Input: part model. Units: mm. Frame: model coordinates. A direction names the side the tool comes from. Round coordinates to 2 decimals unless told otherwise and drop trailing zeros. Write each loop counter-clockwise with the first axis right and the second up, starting at its lowest first coordinate (ties: lowest second). Pieces come first, ordered by that corner, then holes. Notation, with made-up numbers: (39, 87) - (96, 87) arc R15 cw to (96, 91) - close; hole circle Ø11 at (-31.75, 56.25). An arc over 180 degrees is marked (long way). Use one line per item in the form item = value.
```python
from build123d import *

# Parameters (mm, degrees)
SKETCH1_R             = 5
BOSS_EXTRUDE1_DEPTH   = 0.1
BOSS_EXTRUDE1_2_DEPTH = 0.1
BOSS_EXTRUDE1_3_DEPTH = 0.1
BOSS_EXTRUDE1_4_DEPTH = 0.1
BOSS_EXTRUDE2_DEPTH   = 3


with BuildPart() as part:
    # Sketch1 → Boss-Extrude1 (new body)
    with BuildSketch(Plane.XY):
        with Locations((-44.491847198, 44.491847198)):
            Circle(SKETCH1_R)
    extrude(amount=BOSS_EXTRUDE1_DEPTH)



with BuildPart() as body_2:
    # Sketch1 → Boss-Extrude1 2 (new body)
    with BuildSketch(Plane.XY):
        with Locations((44.491847198, 44.491847198)):
            Circle(SKETCH1_R)
    extrude(amount=BOSS_EXTRUDE1_2_DEPTH)


with BuildPart() as body_3:
    # Sketch1 → Boss-Extrude1 3 (new body)
    with BuildSketch(Plane.XY):
        with Locations((44.491847198, -44.491847198)):
            Circle(SKETCH1_R)
    extrude(amount=BOSS_EXTRUDE1_3_DEPTH)


with BuildPart() as body_4:
    # Sketch1 → Boss-Extrude1 4 (new body)
    with BuildSketch(Plane.XY):
        with Locations((-44.491847198, -44.491847198)):
            Circle(SKETCH1_R)
    extrude(amount=BOSS_EXTRUDE1_4_DEPTH)


with BuildPart() as part_1:
    add(part.part)

    add(body_2.part)  # Boss-Extrude2 merges body 2

    add(body_3.part)  # Boss-Extrude2 merges body 3

    add(body_4.part)  # Boss-Extrude2 merges body 4
    # Sketch2 → Boss-Extrude2 (add)
    with BuildSketch(Plane.XY):
        with BuildLine():
            Line((-59.341089603, 40.956313292), (-40.956313292, 59.341089603))
            ThreePointArc((-40.956313292, 59.341089603), (0, 47.170862812), (40.956313292, 59.341089603))
            Line((40.956313292, 59.341089603), (59.341089603, 40.956313292))
            ThreePointArc((59.341089603, 40.956313292), (39.686643359, 0), (59.341089603, -40.956313292))
            Line((59.341089603, -40.956313292), (40.956313292, -59.341089603))
            ThreePointArc((40.956313292, -59.341089603), (0, -47.170862812), (-40.956313292, -59.341089603))
            Line((-40.956313292, -59.341089603), (-59.341089603, -40.956313292))
            ThreePointArc((-59.341089603, -40.956313292), (-39.686643359, 0), (-59.341089603, 40.956313292))
        make_face()
        with BuildLine():
            Line((-32.376492153, 42.376492153), (0, 10))
            Line((0, 10), (32.376492153, 42.376492153))
            ThreePointArc((32.376492153, 42.376492153), (32.490402214, 43.654502905), (31.252682932, 43.99264188))
            ThreePointArc((31.252682932, 43.99264188), (0, 37.170862812), (-31.252682932, 43.99264188))
            ThreePointArc((-31.252682932, 43.99264188), (-32.490402214, 43.654502905), (-32.376492153, 42.376492153))
        make_face(mode=Mode.SUBTRACT)
        with BuildLine():
            Line((-37.410135101, 29.495739933), (-10, 0))
            Line((-10, 0), (-37.410135101, -29.495739933))
            ThreePointArc((-37.410135101, -29.495739933), (-38.724006049, -29.628666123), (-39.024062115, -28.342628566))
            ThreePointArc((-39.024062115, -28.342628566), (-31.907853639, 0), (-39.024062115, 28.342628566))
            ThreePointArc((-39.024062115, 28.342628566), (-38.724006049, 29.628666123), (-37.410135101, 29.495739933))
        make_face(mode=Mode.SUBTRACT)
        with BuildLine():
            Line((10, 0), (37.410135101, -29.495739933))
            ThreePointArc((37.410135101, -29.495739933), (38.724006049, -29.628666123), (39.024062115, -28.342628566))
            ThreePointArc((39.024062115, -28.342628566), (31.907853639, 0), (39.024062115, 28.342628566))
            ThreePointArc((39.024062115, 28.342628566), (38.724006049, 29.628666123), (37.410135101, 29.495739933))
            Line((37.410135101, 29.495739933), (10, 0))
        make_face(mode=Mode.SUBTRACT)
        with BuildLine():
            Line((0, -10), (32.376492153, -42.376492153))
            ThreePointArc((32.376492153, -42.376492153), (32.490402214, -43.654502905), (31.252682932, -43.99264188))
            ThreePointArc((31.252682932, -43.99264188), (0, -37.170862812), (-31.252682932, -43.99264188))
            ThreePointArc((-31.252682932, -43.99264188), (-32.490402214, -43.654502905), (-32.376492153, -42.376492153))
            Line((-32.376492153, -42.376492153), (0, -10))
        make_face(mode=Mode.SUBTRACT)
    extrude(amount=BOSS_EXTRUDE2_DEPTH)


solid = part_1.part
```
(1) First-contact query: pin 1 Ø1 at (y, z) = (7, 2.5) entering from +X; pin 2 Ø8 at (x, y) = (-20, -47) entering from -Z. Flat tips, straight axial feed; report the tip coordinate or a pass-through.
Derived:
pin_1 = 40.23
pin_2 = 0
(2) Cut plane C-C on x = -15.5. Output: boundary loops of the cut face in (y, z).
Derived:
outline = (-48.79, 0) - (-38.79, 0) - (-38.79, 3) - (-48.79, 3) - close; (-25.5, 0) - (-5.92, 0) - (-5.92, 3) - (-25.5, 3) - close; (5.92, 0) - (25.5, 0) - (25.5, 3) - (5.92, 3) - close; (38.79, 0) - (48.79, 0) - (48.79, 3) - (38.79, 3) - close
(3) Access query for faces 4 (the face through (-39.69, -0.66, 1.48)), 5 (the face through (-23.897, 14.954, 1.479)). Directions: +Z, -Z, +X, -X, +Y, -Y. A direction counts if a zero-diameter tool reaches every point of the face in a straight line with its end or side. Return the directions, or none.
Derived:
face_4 = +Z, -Z, -X
face_5 = +Z, -Z
(4) Cut plane D-D on y = 2.5. Output: boundary loops of the cut face in (x, z), then the cut area to 3 significant figures.
Derived:
outline = (-39.75, 0) - (-31.96, 0) - (-31.96, 3) - (-39.75, 3) - close; (-12.32, 0) - (12.32, 0) - (12.32, 3) - (-12.32, 3) - close; (31.96, 0) - (39.75, 0) - (39.75, 3) - (31.96, 3) - close
area = 121 mm^2
(5) Cut plane A-A on z = 0.6. Output: boundary loops of the cut face in (x, y) (1 decimal), then the cut area to 3 significant figures.
Derived:
outline = (-59.3, -41) - (-41, -59.3) arc R75 cw to (41, -59.3) - (59.3, -41) arc R52.5 cw to (59.3, 41) - (41, 59.3) arc R75 cw to (-41, 59.3) - (-59.3, 41) arc R52.5 cw to start; hole (-39, -28.3) arc R1 ccw to (-37.4, -29.5) - (-10, 0) - (-37.4, 29.5) arc R1 ccw to (-39, 28.3) arc R60 cw to start; hole (-32.4, -42.4) arc R1 ccw to (-31.3, -44) arc R75 cw to (31.3, -44) arc R1 ccw to (32.4, -42.4) - (0, -10) - close; hole (-32.4, 42.4) - (0, 10) - (32.4, 42.4) arc R1 ccw to (31.3, 44) arc R75 cw to (-31.3, 44) arc R1 ccw to start; hole (10, 0) - (37.4, -29.5) arc R1 ccw to (39, -28.3) arc R60 cw to (39, 28.3) arc R1 ccw to (37.4, 29.5) - close
area = 6,820 mm^2
(6) Cut plane B-B on y = -15. Output: boundary loops of the cut face in (x, z).
Derived:
outline = (-41.88, 0) - (-33.81, 0) - (-33.81, 3) - (-41.88, 3) - close; (-23.94, 0) - (-5, 0) - (-5, 3) - (-23.94, 3) - close; (5, 0) - (23.94, 0) - (23.94, 3) - (5, 3) - close; (33.81, 0) - (41.88, 0) - (41.88, 3) - (33.81, 3) - close
(7) Material intervals for L1, parallel to Y at x = 19.5, z = 0.15; L2, parallel to X at y = -24, z = 0.8; L3, parallel to X at y = 15, z = 0.45, sorted ascending.
Derived:
L1 = -49.75 to -39.75, -29.5 to -10.22, 10.22 to 29.5, 39.75 to 49.75
L2 = -45.49 to -36.92, -32.3 to -14, 14 to 32.3, 36.92 to 45.49
L3 = -41.88 to -33.81, -23.94 to -5, 5 to 23.94, 33.81 to 41.88
(8) Draft query along Y for faces 1 (the face through (0.607, -47.173, 1.479)), 2 (the face through (-50.3, 50, 1.5)), 3 (the face through (-16, 26, 1)). Return one class per face: released by +Y, released by -Y, zero draft, split by the parting line, or undercut.
Derived:
face_1 = released by -Y
face_2 = released by +Y
face_3 = undercut
